Geometry check sheet. Reference: drawing and pictorial views, mm from the part's lowest x, y, z. Round coordinates to 2 decimals unless told otherwise and drop trailing zeros. Write each loop counter-clockwise with the first axis right and the second up, starting at its lowest first coordinate (ties: lowest second). Pieces come first, ordered by that corner, then holes. Notation, with made-up numbers: M -29,44.5 L -2,44.5 A17 ccw -2,63.5 Z; hole C 45.25,51.5 d5. An arc over 180 degrees is marked long. Use a Markdown table: item, result. Add a question column.
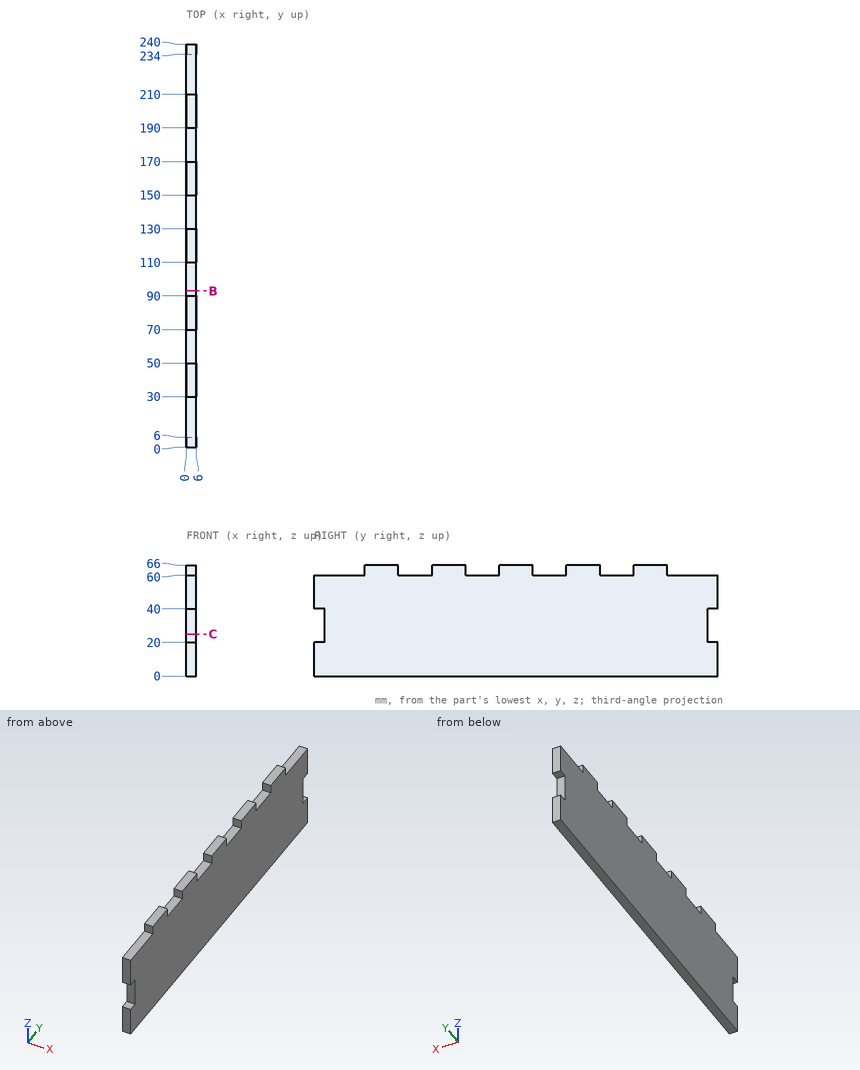
1. Cross-section at B-B on y = 93. Enter the section's corners in (x, z), plus the area to 3 significant figures.
2. Cross-section at C-C on z = 25. Enter the section's corners in (x, y).
3. Scan lines: line 1 along Y through (x, z) = (1.9, 61); line 2 along Z through (x, y) = (2.25, 211.5); line 3 along Y through (x, z) = (5.55, 29). Record each from-to range of solid material in increasing order. Write a range as from..to.
4. Depth check by flat-ended pin: pin 1 Ø1.8 at (x, y) = (3, 237.5) entering from +Z; pin 2 Ø1.8 at (x, z) = (3.5, 32.5) entering from -Y; pin 3 Ø1.8 at (x, z) = (3.5, 62) entering from -Y. Enter the tip coordinate at first touch or a pass-through.
Answer:
| question | item | result |
|---|---|---|
| 1 | outline | M 0,0 L 6,0 L 6,60 L 0,60 Z |
| 1 | area | 360 mm^2 |
| 2 | outline | M 0,6 L 6,6 L 6,234 L 0,234 Z |
| 3 | line 1 | y = 30..50, 70..90, 110..130, 150..170, 190..210 |
| 3 | line 2 | z = 0..60 |
| 3 | line 3 | y = 6..234 |
| 4 | pin 1 | stops at z = 60 |
| 4 | pin 2 | stops at y = 6 |
| 4 | pin 3 | stops at y = 30 |
